Model file for the job. Use its own axes, mm. Face numbers are marked on the shaded views. A direction names the side the tool comes from. Round coordinates to 2 decimals unless told otherwise and drop trailing zeros. Loops run counter-clockwise (first coordinate to the right, second up) from the corner with the lowest first, then second, coordinate; pieces in that order, holes last. Notation, with made-up numbers: M -34,-5.75 L -16,-5.75 A13 ccw -16,13.25 Z; hole C 30.5,11.25 d8. An arc over 180 degrees is marked long. Use a Markdown table: item, result. Add a question column.
Item 1: Saw through at A-A on z = 290. Write the cut outline in (x, y).
Item 2: Wall check: L1, parallel to X at y = 0, z = 155; L2, parallel to Z at x = -8.8, y = 0. Give the ranges that are in metal, low to high. Write a range as from..to.
Item 3: Pin check, flat tips, straight feed: P1, Ø1.5, axis at y = 3.5, z = 192, coming from the -X side; P2, Ø6, axis at x = -3, z = 260, coming from the -Y side; P3, Ø1, axis at y = 6, z = 252.5, coming from the +X side; P4, Ø9.5, axis at y = 0, z = 290, coming from the -X side. Stop position of each tip, or through.
Item 4: Saw through at C-C on z = 22. Write the cut outline in (x, y), then the cut area to 3 significant figures.
Item 5: Tool access for the marked faces 1 and 2: list every direction of +Z, -Z, +X, -X, +Y, -Y with a clear straight run to the whole face (end or side of a thin tool).
Item 6: Saw through at B-B on y = 0. Give the number of separate pieces and of enclosed holes in the cut face, then the cut area to 3 significant figures.
Item 7: Saw through at D-D on z = 74. Write the cut outline in (x, y), then the cut area to 3 significant figures.
```python
from build123d import *

# Parameters (mm, degrees)
F0_R          = 9.7
F1_DEPTH      = 268
F2_R          = 8.5
F3_DEPTH      = 33
F5_R          = 7.5
F6_DEPTH      = 36.4
F7_R          = 8.5
F8_DEPTH      = 267
F4_R          = 3
F9_DEPTH      = 25
F9_DEPTH_BACK = 25


# Not quite as in the source:
# - a fillet or chamfer that OpenCascade refuses, or shapes differently, is made with other operations: its cross-section is extruded or revolved along the edge and cut away or added


with BuildPart() as f1:
    # F0 (on Top) → F1 (new body)
    with BuildSketch(Plane.XY):
        Circle(F0_R)
    extrude(amount=F1_DEPTH)

    # F2 (on face) → F3 (join)
    with BuildSketch(Plane.XY.offset(268)):
        Circle(F2_R)
    extrude(amount=F3_DEPTH)

    # F5 (on face) → F6 (cut)
    with BuildSketch(Plane.XY.offset(301)):
        Circle(F5_R)
    extrude(amount=-F6_DEPTH, mode=Mode.SUBTRACT)

    # F7 (on face) → F8 (cut)
    with BuildSketch(Plane(origin=(0, 0, 0), x_dir=(1, 0, 0), z_dir=(0, 0, -1))):
        Circle(F7_R)
    extrude(amount=-F8_DEPTH, mode=Mode.SUBTRACT)

    # F4 (on Right) → F9 (cut, two sides)
    with BuildSketch(Plane.YZ) as f9_sk:
        with Locations((0, 22)):
            Circle(F4_R)
        with Locations((0, 290)):
            Circle(F4_R)
    extrude(amount=-F9_DEPTH, mode=Mode.SUBTRACT)
    extrude(f9_sk.sketch, amount=F9_DEPTH_BACK, mode=Mode.SUBTRACT)

    # F10: fillet of radius 5 on 1 edges, made by hand

    # F10_s1 → F10_t2 (revolve, cut)
    with BuildSketch(Plane.XZ):
        with BuildLine():
            add(Edge.make_bspline(
                [(9.7, 264.7503846381), (9.7, 266.5967570028), (8.5, 268)],
                knots=[0, 0, 0, 1, 1, 1], degree=2, weights=[1, 1, 1]))
            Line((8.5, 268), (8.576, 268.0649923072))
            ThreePointArc((8.576, 268.0649923072), (9.1, 268.1), (9.7, 268.1))
            Line((9.7, 268.1), (9.8, 268))
            Line((9.8, 268), (9.8, 264.7503846381))
            Line((9.8, 264.7503846381), (9.7, 264.7503846381))
        make_face()
    revolve(axis=Axis((0, 0, 268), (0, 0, 1)), mode=Mode.SUBTRACT)


solid = f1.part
```
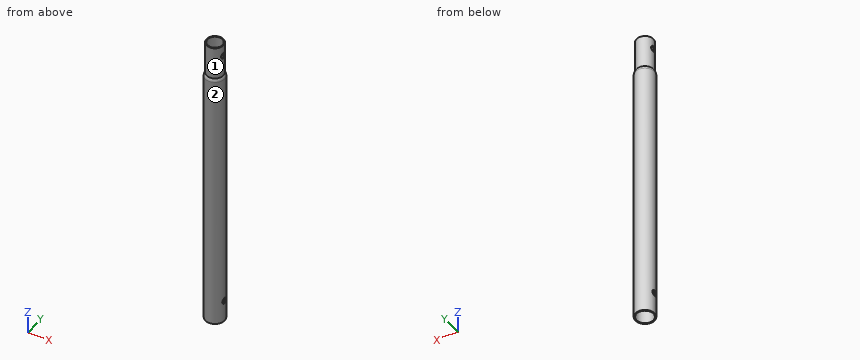
Entries:
| question | item | result |
|---|---|---|
| 1 | outline | M -7.95,-3 A8.5 ccw 7.95,-3 L 6.87,-3 A7.5 cw -6.87,-3 Z; M -7.95,3 L -6.87,3 A7.5 cw 6.87,3 L 7.95,3 A8.5 ccw Z |
| 2 | L1 | -9.7..-8.5, 8.5..9.7 |
| 2 | L2 | 0..19, 25..267.62 |
| 3 | P1 | x = -9.3 |
| 3 | P2 | y = -9.7 |
| 3 | P3 | x = 7.99 |
| 3 | P4 | x = -8.5 |
| 4 | outline | M -9.22,-3 A9.7 ccw 9.22,-3 L 7.95,-3 A8.5 cw -7.95,-3 Z; M -9.22,3 L -7.95,3 A8.5 cw 7.95,3 L 9.22,3 A9.7 ccw Z |
| 4 | area | 53.9 mm2 |
| 5 | face 1 | +Z |
| 5 | face 2 | +Z, -Z |
| 6 | separate pieces | 6 |
| 6 | enclosed holes | 0 |
| 6 | area | 682 mm2 |
| 7 | outline | C 0,0 d19.4; hole C 0,0 d17 |
| 7 | area | 68.6 mm2 |
